Geometry: final body of the model. Coordinates: model frame, mm. Face numbers are marked on the shaded views. A direction names the side the tool comes from. Round coordinates to 2 decimals unless told otherwise and drop trailing zeros. Loops run counter-clockwise (first coordinate to the right, second up) from the corner with the lowest first, then second, coordinate; pieces in that order, holes last. Notation, with made-up numbers: (-2, -14) - (48, -14) arc R13 cw to (48, 5) - close; hole circle Ø10 at (-19.5, -20). An arc over 180 degrees is marked (long way). Answer as CSV lines item,"result".
from build123d import *

# Parameters (mm, degrees)
SKETCH1_R               = 4.75
SKETCH1_R_2             = 1.95
BOSS_EXTRUDE1_DEPTH     = 35
CUT_EXTRUDE1_DEPTH      = 36.638813112
CUT_EXTRUDE1_DEPTH_BACK = 36.638813112
SKETCH2_W               = 7.1
SKETCH2_H               = 3.3


with BuildPart() as part:
    # Sketch1 → Boss-Extrude1 (new body)
    with BuildSketch(Plane(origin=(0, 0, 0), x_dir=(1, 0, 0), z_dir=(0, 1, 0))):
        with Locations(Location((0, 0, 0), (0, 0, 270))):
            Circle(SKETCH1_R)
        with Locations(Location((0, 0, 0), (0, 0, 270))):
            Circle(SKETCH1_R_2, mode=Mode.SUBTRACT)
    extrude(amount=BOSS_EXTRUDE1_DEPTH)

    # Sketch2 → Cut-Extrude1 (cut, two sides: drawn at the far end of the back side and taken through both)
    with BuildSketch(Plane.XY.offset(-CUT_EXTRUDE1_DEPTH_BACK)):
        with Locations((0, 30)):
            Rectangle(SKETCH2_W, SKETCH2_H)
        with Locations((0, 5)):
            Rectangle(SKETCH2_W, SKETCH2_H)
    extrude(amount=CUT_EXTRUDE1_DEPTH + CUT_EXTRUDE1_DEPTH_BACK, mode=Mode.SUBTRACT)


solid = part.part
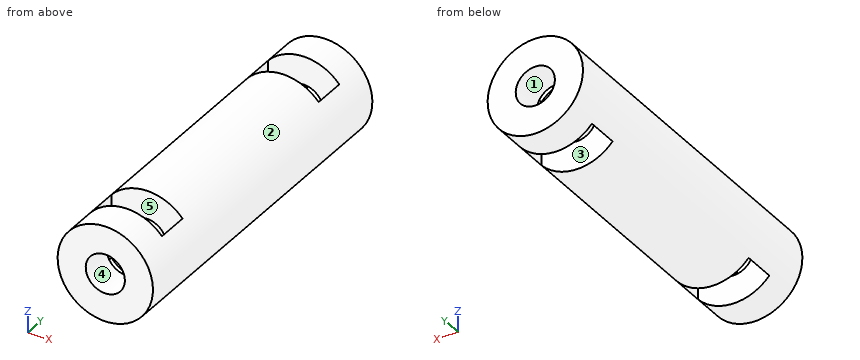
(1) Pin query (flat end, axial travel): P1, Ø1, axis at y = 30, z = -1.5, coming from the -X side; P2, Ø5, axis at x = 3.5, y = 7, coming from the -Z side. Return the tip coordinate at first contact, or that it passes through.
Findings below:
P1,"x = -4.64"
P2,"z = -4.64"
(2) Material intervals for line 1 along Y through (x, z) = (2.5, 0.25); line 2 along X through (y, z) = (32.4, 0), sorted ascending.
Findings below:
line 1,"0 to 3.35, 6.65 to 28.35, 31.65 to 35"
line 2,"-4.75 to -1.95, 1.95 to 4.75"
(3) Section B-B (x = 0). Output: boundary loops of the cut face in (y, z).
Findings below:
outline,"(0, -4.75) - (3.35, -4.75) - (3.35, -1.95) - (0, -1.95) - close; (0, 1.95) - (3.35, 1.95) - (3.35, 4.75) - (0, 4.75) - close; (6.65, -4.75) - (28.35, -4.75) - (28.35, -1.95) - (6.65, -1.95) - close; (6.65, 1.95) - (28.35, 1.95) - (28.35, 4.75) - (6.65, 4.75) - close; (31.65, -4.75) - (35, -4.75) - (35, -1.95) - (31.65, -1.95) - close; (31.65, 1.95) - (35, 1.95) - (35, 4.75) - (31.65, 4.75) - close"
(4) Draft query along Z for the marked faces 1, 2 and 3. Return one class per face: pulls with the +Z half, pulls with the -Z half, needs draft (parallel to the pull), parting line crosses it, or undercut.
Findings below:
face 1,"undercut"
face 2,"parting line crosses it"
face 3,"needs draft"
(5) Section C-C (y = 10). Output: boundary loops of the cut face in (x, z), and give its area (3 significant figures).
Findings below:
outline,"circle Ø9.5 at (0, 0); hole circle Ø3.9 at (0, 0)"
area,"58.9 mm2"
(6) Section D-D (x = 2.5). Output: boundary loops of the cut face in (y, z), and give its area (3 significant figures).
Findings below:
outline,"(0, -4.04) - (3.35, -4.04) - (3.35, 4.04) - (0, 4.04) - close; (6.65, -4.04) - (28.35, -4.04) - (28.35, 4.04) - (6.65, 4.04) - close; (31.65, -4.04) - (35, -4.04) - (35, 4.04) - (31.65, 4.04) - close"
area,"229 mm2"
(7) Access query for the marked faces 4 and 5. Directions: +Z, -Z, +X, -X, +Y, -Y. A direction counts if a zero-diameter tool reaches every point of the face in a straight line with its end or side. Return the directions, or none.
Findings below:
face 4,"+Y, -Y"
face 5,"+Z, -Z"
(8) Section A-A (z = 0). Output: boundary loops of the cut face in (x, y).
Findings below:
outline,"(-4.75, 0) - (-1.95, 0) - (-1.95, 3.35) - (-3.55, 3.35) - (-3.55, 6.65) - (-1.95, 6.65) - (-1.95, 28.35) - (-3.55, 28.35) - (-3.55, 31.65) - (-1.95, 31.65) - (-1.95, 35) - (-4.75, 35) - close; (1.95, 0) - (4.75, 0) - (4.75, 35) - (1.95, 35) - (1.95, 31.65) - (3.55, 31.65) - (3.55, 28.35) - (1.95, 28.35) - (1.95, 6.65) - (3.55, 6.65) - (3.55, 3.35) - (1.95, 3.35) - close"
